Check sheet for the modelled part. Datum: model origin and axes. Units: mm. Face numbers are marked on the shaded views. A direction names the side the tool comes from. Round coordinates to 2 decimals unless told otherwise and drop trailing zeros. Write each loop counter-clockwise with the first axis right and the second up, starting at its lowest first coordinate (ties: lowest second). Pieces come first, ordered by that corner, then holes. Notation, with made-up numbers: (75.25, -21) -> (127.25, -21) arc R28 cw to (127.25, 6) -> close; hole circle Ø6 at (-38.75, -20.5). An arc over 180 degrees is marked (long way). Use one line per item in the form item = value. Start each with the question number.
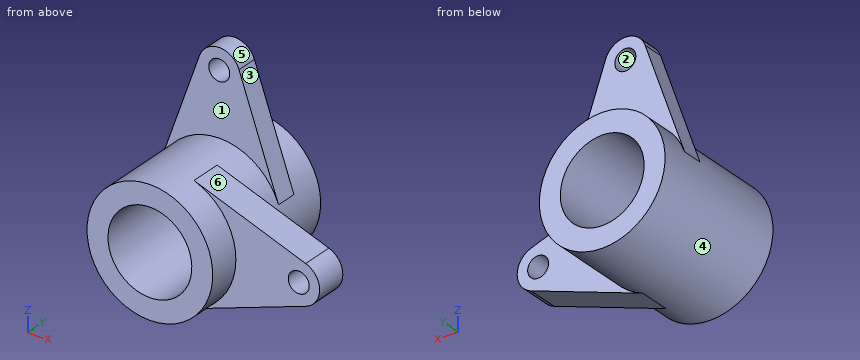
```python
from build123d import *

# Parameters (mm, degrees)
SKETCH2_R           = 30
SKETCH2_R_2         = 20
BOSS_EXTRUDE1_DEPTH = 70
SKETCH4_R           = 5
BOSS_EXTRUDE2_DEPTH = 15
SKETCH5_R           = 5
BOSS_EXTRUDE3_DEPTH = 10


with BuildPart() as part:
    # Sketch2 → Boss-Extrude1 (new body)
    with BuildSketch(Plane(origin=(0, 0, 0), x_dir=(1, 0, 0), z_dir=(0, 1, 0))):
        with Locations(Location((0, 0, 0), (0, 0, 270))):
            Circle(SKETCH2_R)
        with Locations(Location((0, 0, 0), (0, 0, 270))):
            Circle(SKETCH2_R_2, mode=Mode.SUBTRACT)
    extrude(amount=BOSS_EXTRUDE1_DEPTH)

    # Sketch4 → Boss-Extrude2 (add)
    with BuildSketch(Plane(origin=(0, 15, 0), x_dir=(1, 0, 0), z_dir=(0, 1, 0))):
        with BuildLine():
            Line((63.333333333, 9.428090416), (10, 28.284271247))
            ThreePointArc((10, 28.284271247), (30, 0), (10, -28.284271247))
            Line((10, -28.284271247), (63.333333333, -9.428090416))
            ThreePointArc((63.333333333, -9.428090416), (70, 0), (63.333333333, 9.428090416))
        make_face()
        with Locations(Location((60, 0, 0), (0, 0, 270))):
            Circle(SKETCH4_R, mode=Mode.SUBTRACT)
    extrude(amount=BOSS_EXTRUDE2_DEPTH)

    # Sketch5 → Boss-Extrude3 (add)
    with BuildSketch(Plane(origin=(0, 45, 0), x_dir=(1, 0, 0), z_dir=(0, 1, 0))):
        with BuildLine():
            Line((-9.428090416, -63.333333333), (-28.284271247, -10))
            ThreePointArc((-28.284271247, -10), (0, -30), (28.284271247, -10))
            Line((28.284271247, -10), (9.428090416, -63.333333333))
            ThreePointArc((9.428090416, -63.333333333), (0, -70), (-9.428090416, -63.333333333))
        make_face()
        with Locations(Location((0, -60, 0), (0, 0, 270))):
            Circle(SKETCH5_R, mode=Mode.SUBTRACT)
    extrude(amount=BOSS_EXTRUDE3_DEPTH)


solid = part.part
```
1. Depth check by flat-ended pin: pin 1 (8 mm diameter, centred on x = 10, z = 8.5, fed in from +Y); pin 2 (12 mm diameter, centred on x = 31, y = 25, fed in from -Z); pin 3 (5 mm diameter, centred on x = 6, y = 23, fed in from -Z); pin 4 (17 mm diameter, centred on x = 39.5, z = -8, fed in from -Y). Enter the tip coordinate at first touch or a pass-through.
2. Mould release check, pull along X, two halves, no side actions. Record for the marked faces 1, 2 and 3: +X half, -X half, draft (parallel to the pull), parting line (faces both ways), or undercut.
3. Sectioned sample at D-D (y = 17.5). Enter the section's corners in (x, z), and give its area (3 significant figures).
4. Sectioned sample at B-B (z = 0). Enter the section's corners in (x, y), and give its area (3 significant figures).
5. Scan lines: probe 1 along X at (y, z) = (28, 0); probe 2 along X at (y, z) = (46, 0); probe 3 along Y at (x, z) = (25, 17). Record each from-to range of solid material in increasing order.
6. Sectioned sample at A-A (x = 0). Enter the section's corners in (y, z), and give its area (3 significant figures).
7. Tool access check on the marked faces 4, 5 and 6. Record the directions out of +Z, -Z, +X, -X, +Y, -Y that give a thin tool (end or side, any length) a straight path to the whole face; none if there is none.
8. Sectioned sample at C-C (x = -12). Enter the section's corners in (y, z), and give its area (4 significant figures).
Returned:
q1.pin_1 = through
q1.pin_2 = -22.98
q1.pin_3 = -29.8
q1.pin_4 = 15
q2.face_1 = draft
q2.face_2 = undercut
q2.face_3 = +X half
q3.outline = (10, -28.28) -> (63.33, -9.43) arc R10 ccw to (63.33, 9.43) -> (10, 28.28) arc R30 ccw (long way) to start; hole circle Ø40 at (0, 0); hole circle Ø10 at (60, 0)
q3.area = 2,770 mm^2
q4.outline = (-30, 0) -> (-20, 0) -> (-20, 70) -> (-30, 70) -> close; (20, 0) -> (30, 0) -> (30, 15) -> (55, 15) -> (55, 30) -> (30, 30) -> (30, 70) -> (20, 70) -> close; (65, 15) -> (70, 15) -> (70, 30) -> (65, 30) -> close
q4.area = 1,850 mm^2
q5.probe_1 = -30 to -20, 20 to 55, 65 to 70
q5.probe_2 = -30 to -20, 20 to 30
q5.probe_3 = 15 to 30, 45 to 55
q6.outline = (0, -30) -> (70, -30) -> (70, -20) -> (0, -20) -> close; (0, 20) -> (70, 20) -> (70, 30) -> (55, 30) -> (55, 55) -> (45, 55) -> (45, 30) -> (0, 30) -> close; (45, 65) -> (55, 65) -> (55, 70) -> (45, 70) -> close
q6.area = 1,700 mm^2
q7.face_4 = none
q7.face_5 = +Z, +Y, -Y
q7.face_6 = +Z, +X, -Y
q8.outline = (0, -27.5) -> (70, -27.5) -> (70, -16) -> (0, -16) -> close; (0, 16) -> (70, 16) -> (70, 27.5) -> (55, 27.5) -> (55, 56.06) -> (45, 56.06) -> (45, 27.5) -> (0, 27.5) -> close
q8.area = 1,895 mm^2
